The model under review builds one solid part; all positions refer to its coordinate system, in mm. A direction names the side the tool comes from. Round coordinates to 2 decimals unless told otherwise and drop trailing zeros. Loops run counter-clockwise (first coordinate to the right, second up) from the corner with the lowest first, then second, coordinate; pieces in that order, holes last. Notation, with made-up numbers: (16.25, 3.5) -> (57.25, 3.5) arc R19 cw to (57.25, 13.5) -> close; hole circle Ø6 at (-39, -6.75). An arc over 180 degrees is marked (long way). Use a Markdown table: item, result. Add a question column.
1) Consider section B-B on z = 10. Give the boundary of the cut face in (x, y).
2) Consider section C-C on y = 132. Give the boundary of the cut face in (x, z).
3) Insertion check: pin 1 (3 mm diameter, centred on x = 3.5, z = 13, fed in from +Y); pin 2 (1.5 mm diameter, centred on x = 3, z = 8, fed in from +Y). Each pin has a flat end and moves straight along its axis. Give the tip position at first contact, or say it passes through.
4) Consider section A-A on y = 30. Give the boundary of the cut face in (x, z).
5) Wall thickness on probe 1 along Z at (x, y) = (-2, 218); probe 2 along Y at (x, z) = (0, 11.75); probe 3 along X at (y, z) = (28, 7.25): over which ranges is each line inside the solid? List them lowest first.
6) For faces 1 (the cylindrical face through (0.33, 27.52, 9.93)), 2 (the flat face through (0, 138, -5)), list the 3-axis set-ups (+Z, -Z, +X, -X, +Y, -Y) from which the entire face can be reached by the end or side of a thin tool; tool diameter is ignored.
from build123d import *

# Parameters (mm, degrees)
SKETCH_1_W      = 10
SKETCH_1_H      = 10
EXTRUDE_1_DEPTH = 280
SKETCH_2_R      = 2.5
EXTRUDE_2_DEPTH = 10
SKETCH_3_W      = 5.326066841
SKETCH_3_H      = 0.31329805
EXTRUDE_3_DEPTH = 0.1


with BuildPart() as part:
    # 草图1 → 凸台-拉伸1 (new body)
    with BuildSketch(Plane(origin=(0, 0, 0), x_dir=(1, 0, 0), z_dir=(0, 1, 0))):
        Rectangle(SKETCH_1_W, SKETCH_1_H)
    extrude(amount=EXTRUDE_1_DEPTH)

    # 草图2 → 凸台-拉伸2 (add)
    with BuildSketch(Plane.XY.offset(5)):
        with Locations(Location((0, 30, 0), (0, 0, 180))):
            Circle(SKETCH_2_R)
    extrude(amount=EXTRUDE_2_DEPTH)

    # 草图3 → 凸台-拉伸3 (add)
    with BuildSketch(Plane.XY.offset(5)):
        with Locations((-2.223790566, 102.242298207)):
            Rectangle(SKETCH_3_W, SKETCH_3_H)
    extrude(amount=EXTRUDE_3_DEPTH)


solid = part.part
Result set:
| question | item | result |
|---|---|---|
| 1 | outline | circle Ø5 at (0, 30) |
| 2 | outline | (-5, -5) -> (5, -5) -> (5, 5) -> (-5, 5) -> close |
| 3 | pin 1 | y = 31.5 |
| 3 | pin 2 | y = 31.09 |
| 4 | outline | (-5, -5) -> (5, -5) -> (5, 5) -> (2.5, 5) -> (2.5, 15) -> (-2.5, 15) -> (-2.5, 5) -> (-5, 5) -> close |
| 5 | probe 1 | -5 to 5 |
| 5 | probe 2 | 27.5 to 32.5 |
| 5 | probe 3 | -1.5 to 1.5 |
| 6 | face 1 | +Z |
| 6 | face 2 | -Z, +X, -X, +Y, -Y |
